Part model, mm, in its own coordinate system. Face numbers are marked on the shaded views. A direction names the side the tool comes from. Coordinates: 2 decimals unless noted, no trailing zeros. Write each loop counter-clockwise with the first axis right and the second up, starting at its lowest first coordinate (ties: lowest second). Pieces come first, ordered by that corner, then holes. Notation, with made-up numbers: (42, -26.5) -> (50, -26.5) arc R26 ccw to (50, 5.5) -> close; hole circle Ø6 at (87.25, 89.5). An arc over 180 degrees is marked (long way). Write item = value, one per line.
from build123d import *

# Parameters (mm, degrees)
BOSS_EXTRUDE1_DEPTH        = 7.9375
F_2_5MM_DOWEL_HOLE1_REACH  = 85.992
F_2_5MM_DOWEL_HOLE1_BORE_R = 1.25
CIRPATTERN1_START          = -22.212933302
CIRPATTERN1_DEPTH          = 57.137933384
CIRPATTERN1_START_2        = -34.9250001
CIRPATTERN1_2_OUTLINE_R    = 1.25
CIRPATTERN1_2_DEPTH        = 12.735179899
BOSS_EXTRUDE2_START        = 1.27
BOSS_EXTRUDE2_DEPTH        = 1.27


# Read off the part's stored shape, not the designer's step: CirPattern1
with BuildPart() as part:
    # Sketch1 → Boss-Extrude1 (new, symmetric)
    with BuildSketch(Plane(origin=(0, 0, 0), x_dir=(1, 0, 0), z_dir=(0, 1, 0))):
        with BuildLine():
            Line((-0.762, 34.916686283), (-0.762, 22.211933302))
            ThreePointArc((-0.762, 22.211933302), (0, -22.225), (0.762, 22.211933302))
            Line((0.762, 22.211933302), (0.762, 34.916686283))
            ThreePointArc((0.762, 34.916686283), (0, -34.925), (-0.762, 34.916686283))
        make_face()
    extrude(amount=BOSS_EXTRUDE1_DEPTH, both=True)

    # Sketch2 → Cut-Revolve1 (revolve, cut)
    with BuildSketch(Plane(origin=(0, 0, 0), x_dir=(1, 0, 0), z_dir=(0, 1, 0)), mode=Mode.PRIVATE) as cut_revolve1_sk:
        Polygon((-22.683703898, 26.5557), (0.762, 26.5557), (0.762, 26.0223), (5.329933657, 26.0223), (5.329933657, 23.8125), (25.548394641, 23.8125), (25.548394641, 28.575), (-22.683703898, 28.575), align=None)
    revolve(cut_revolve1_sk.sketch.rotate(Axis((-22.683703898, 0, -28.575), (-1, 0, 0)), 180), axis=Axis((-22.683703898, 0, -28.575), (-1, 0, 0)), mode=Mode.SUBTRACT)

    # Ø2.5mm Dowel Hole1 bore (on position points) → Ø2.5mm Dowel Hole1 (cut, up to next)
    with BuildSketch(Plane(origin=(30.245937227, 0, -17.4625), x_dir=(0.5, 0, 0.866025403784), z_dir=(0.866025403784, 0, -0.5)), mode=Mode.PRIVATE) as f_2_5mm_dowel_hole1_sk1:
        Circle(F_2_5MM_DOWEL_HOLE1_BORE_R)
    f_2_5mm_dowel_hole1_tool1 = extrude(f_2_5mm_dowel_hole1_sk1.sketch, amount=-F_2_5MM_DOWEL_HOLE1_REACH, mode=Mode.PRIVATE) & part.part
    add(f_2_5mm_dowel_hole1_tool1.solids().sort_by_distance((30.245937, 0, -17.4625))[0], mode=Mode.SUBTRACT)

    # CirPattern1 outline → CirPattern1 (cut)
    with BuildSketch(Plane.XY.offset(CIRPATTERN1_START)):
        with BuildLine():
            ThreePointArc((-0.762, -0.990886472), (1.25, 0), (-0.762, 0.990886472))
            ThreePointArc((-0.762, 0.990886472), (-1.25, 0), (-0.762, -0.990886472))
        make_face()
    extrude(amount=CIRPATTERN1_DEPTH, mode=Mode.SUBTRACT)

    # CirPattern1 2 outline → CirPattern1 2 (cut)
    with BuildSketch(Plane(origin=(0, 0, 0), x_dir=(0.500000000000004, 0, -0.8660254037844363), z_dir=(0.8660254037844363, 0, 0.5000000000000042)).offset(CIRPATTERN1_START_2)):
        Circle(CIRPATTERN1_2_OUTLINE_R)
    extrude(amount=CIRPATTERN1_2_DEPTH, mode=Mode.SUBTRACT)

    # Sketch4 → Boss-Extrude2 (add)
    with BuildSketch(Plane(origin=(0, 7.9375, 0), x_dir=(1, 0, 0), z_dir=(0, 1, 0)).offset(BOSS_EXTRUDE2_START)):
        with BuildLine():
            Line((0.762, 34.916686283), (0.762, 19.670246084))
            ThreePointArc((0.762, 19.670246084), (0, -19.685), (-0.762, 19.670246084))
            Line((-0.762, 19.670246084), (-0.762, 34.916686283))
            ThreePointArc((-0.762, 34.916686283), (0, -34.925), (0.762, 34.916686283))
        make_face()
    extrude(amount=-BOSS_EXTRUDE2_DEPTH)


solid = part.part
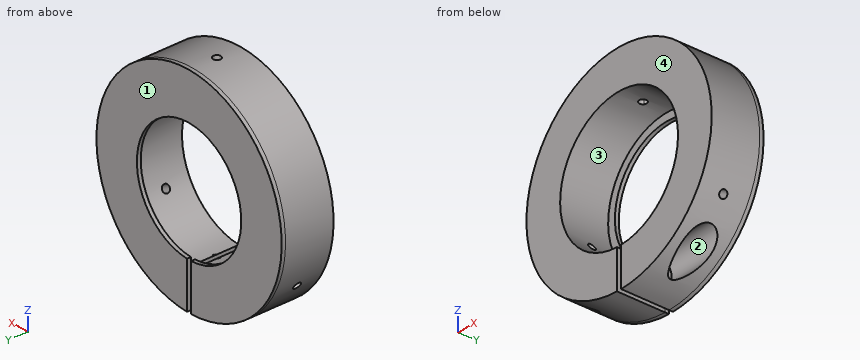
Q1. Which spindle directions (+Z, -Z, +X, -X, +Y, -Y) get a long thin tool onto all of the face, cutting with end or side? Do the marked faces 1 and 2. Say none if no direction does.
Model answer:
face_1 = +Z, -Z, +X, -X, +Y
face_2 = +X
Q2. Probe line 1 (Y direction, x = 28, z = -16); line 2 (X direction, y = 6.25, z = 1); line 3 (Z direction, x = -12, y = 4.5). List the from-to ranges inside material, lowest first. Write a range as from..to.
Model answer:
line_1 = -7.94..-1.24, 1.24..9.21
line_2 = -34.91..-22.2, 22.2..34.91
line_3 = -32.8..-18.71, 18.71..32.8
Q3. Saw through at C-C on y = 0. Count the separate pieces of the cut face and the enclosed holes in it, and give its area (3 significant figures).
Model answer:
separate_pieces = 6
enclosed_holes = 0
area = 1,930 mm²
Q4. Pin check, flat tips, straight feed: pin 1 (1 mm diameter, centred on y = 0, z = -16, fed in from +X); pin 2 (7.5 mm diameter, centred on y = 3.5, z = -27.5, fed in from -X); pin 3 (1 mm diameter, centred on y = 9, z = -28.5, fed in from +X); pin 4 (12 mm diameter, centred on x = 25, z = -24.5, fed in from -Y). Stop position of each tip, or through.
Model answer:
pin_1 = 31.3
pin_2 = -25.61
pin_3 = 20.87
pin_4 = -7.94
Q5. Saw through at B-B on z = 0. Give the cut face in (x, y) (1 decimal).
Model answer:
outline = (-34.9, -7.9) -> (-22.2, -7.9) -> (-22.2, 7.9) -> (-19.7, 7.9) -> (-19.7, 9.2) -> (-34.9, 9.2) -> close; (19.7, 7.9) -> (22.2, 7.9) -> (22.2, -7.9) -> (34.9, -7.9) -> (34.9, 9.2) -> (19.7, 9.2) -> close
Q6. Saw through at A-A on x = -13.5. Give the cut face in (y, z) (1 decimal).
Model answer:
outline = (-7.9, -32.2) -> (9.2, -32.2) -> (9.2, -14.3) -> (7.9, -14.3) -> (7.9, -17.7) -> (-7.9, -17.7) -> close; (-7.9, 17.7) -> (7.9, 17.7) -> (7.9, 14.3) -> (9.2, 14.3) -> (9.2, 32.2) -> (-7.9, 32.2) -> close; hole circle Ø4 at (0, -28.6)
Q7. Saw through at D-D on z = -28.5. Give the cut face in (x, y).
Model answer:
outline = (-20.19, -7.94) -> (-0.76, -7.94) -> (-0.76, -2.02) -> (-20.19, -2.02) -> close; (-20.19, 2.02) -> (-0.76, 2.02) -> (-0.76, 9.21) -> (-20.19, 9.21) -> close; (0.76, -7.94) -> (20.19, -7.94) -> (20.19, -4.76) -> (5.33, -4.76) -> (5.33, -2.55) -> (0.76, -2.55) -> close; (0.76, 2.55) -> (5.33, 2.55) -> (5.33, 4.76) -> (20.19, 4.76) -> (20.19, 9.21) -> (0.76, 9.21) -> close
Q8. Mould opens along X. For the marked faces 3 and 4 say: released by +X, released by -X, zero draft, split by the parting line, or undercut.
Model answer:
face_3 = undercut
face_4 = zero draft
